Part model, mm, in its own coordinate system. A direction names the side the tool comes from. Give positions to 0.01 mm unless a question says otherwise; leave off trailing zeros. Write each loop counter-clockwise with the first axis right and the second up, starting at its lowest first coordinate (ties: lowest second). Pieces come first, ordered by that corner, then holes. Notation, with made-up numbers: M 19.25,33.25 L 42.25,33.25 A20 cw 42.25,71.25 Z; hole C 43.5,-15 d5. An arc over 180 degrees is marked long. Use CSV: the item, a comma, the result in double quotes. Start each with the question number.
1. Drill centre lines: line 1 along Y through (x, z) = (2, 1.2); line 2 along X through (y, z) = (-8, 1.7); line 3 along X through (y, z) = (14.5, 1.85). Where is each one in solid material? Low to high. Write a range as from..to.
2. Band-saw the part on A-A, the plane z = 1.9. List the corners of the cut face in (x, y), then the cut area to 3 significant figures.
3. Band-saw the part on B-B, the plane y = 1.5. List the corners of the cut face in (x, z).
4. Band-saw the part on C-C, the plane x = 0.5. List the corners of the cut face in (y, z).
5. Drop flat-ended pins along their axis: pin 1 Ø1.5 at (y, z) = (8.5, 0.5) entering from +X; pin 2 Ø1 at (y, z) = (4, 2) entering from -X; pin 3 Ø1.5 at (x, z) = (4.5, 1) entering from +Y. Give the stop position or say it passes through.
6. 3-axis set-ups, long thin cutter, end or side, ignore diameter. For faces 1 (the face through (-22, -10.5, 1)), 2 (the face through (-3.5, 12, 1)), 3 (the face through (-24.3, 13, 1)): which of +Z, -Z, +X, -X, +Y, -Y reach the whole face in a straight line?
7. Mould opens along Y. For faces 4 (the face through (-22, 10.5, 1)), 5 (the face through (18.64, 9.6, 1.48)), 6 (the face through (19.5, -3, 1)) say: pulls with the +Y half, pulls with the -Y half, needs draft (parallel to the pull), parting line crosses it, or undercut.
from build123d import *

# Parameters (mm, degrees)
SKETCH_1_W      = 4.8
SKETCH_1_H      = 5
EXTRUDE_1_DEPTH = 3
FILLET_1_R      = 0.5


with BuildPart() as part:
    # Эскиз1 → Бобышка-Вытянуть1 (new body)
    with BuildSketch(Plane.XY):
        with BuildLine():
            Line((-4.5, 15.5), (-19.5, 15.5))
            Line((-19.5, 15.5), (-19.5, 10.5))
            Line((-19.5, 10.5), (-19.5, -10.5))
            Line((-19.5, -10.5), (-19.5, -15.5))
            Line((-19.5, -15.5), (16.5, -15.5))
            ThreePointArc((16.5, -15.5), (18.621320344, -14.621320344), (19.5, -12.5))
            Line((19.5, -12.5), (19.5, 7.5))
            ThreePointArc((19.5, 7.5), (18.621320344, 9.621320344), (16.5, 10.5))
            Line((16.5, 10.5), (-3.5, 10.5))
            Line((-3.5, 10.5), (-3.5, 14.5))
            ThreePointArc((-3.5, 14.5), (-3.792893219, 15.207106781), (-4.5, 15.5))
        make_face()
        with Locations((-21.9, -13)):
            Rectangle(SKETCH_1_W, SKETCH_1_H)
        with Locations((-21.9, 13)):
            Rectangle(SKETCH_1_W, SKETCH_1_H)
    extrude(amount=EXTRUDE_1_DEPTH)

    # Скругление1
    fillet_1_edges = [part.edges().sort_by_distance(p)[0] for p in [
        (-24.3, -15.5, 1.5),
        (-24.3, -10.5, 1.5),
        (-24.3, 15.5, 1.5),
        (-24.3, 10.5, 1.5),
    ]]
    fillet(fillet_1_edges, radius=FILLET_1_R)


solid = part.part
Output:
1,line 1,"y = -15.5..10.5"
1,line 2,"x = -19.5..19.5"
1,line 3,"x = -24.3..-3.5"
2,outline,"M -24.3,-15 A0.5 ccw -23.8,-15.5 L 16.5,-15.5 A3 ccw 19.5,-12.5 L 19.5,7.5 A3 ccw 16.5,10.5 L -3.5,10.5 L -3.5,14.5 A1 ccw -4.5,15.5 L -23.8,15.5 A0.5 ccw -24.3,15 L -24.3,11 A0.5 ccw -23.8,10.5 L -19.5,10.5 L -19.5,-10.5 L -23.8,-10.5 A0.5 ccw -24.3,-11 Z"
2,area,"1,140 mm²"
3,outline,"M -19.5,0 L 19.5,0 L 19.5,3 L -19.5,3 Z"
4,outline,"M -15.5,0 L 10.5,0 L 10.5,3 L -15.5,3 Z"
5,pin 1,"stops at x = 19.49"
5,pin 2,"stops at x = -19.5"
5,pin 3,"stops at y = 10.5"
6,face 1,"+Z, -Z, -X"
6,face 2,"+Z, -Z, +X, +Y"
6,face 3,"+Z, -Z, -X, +Y, -Y"
7,face 4,"undercut"
7,face 5,"pulls with the +Y half"
7,face 6,"needs draft"
